from build123d import *

# Parameters (mm, degrees)
CYLINDER189_R               = 5
CYLINDER189_DEPTH           = 8
CYLINDER189_ROLL_ANGLE      = 90
BOX001027045139_W           = 21
BOX001027045139_H           = 10
BOX001027045139_DEPTH       = 28
BOX001027045139_PITCH_ANGLE = 45
BOX001027045138_W           = 21
BOX001027045138_H           = 10
BOX001027045138_DEPTH       = 28
BOX001027045137_W           = 21
BOX001027045137_H           = 8
BOX001027045137_DEPTH       = 28


with BuildPart() as screw_bump_top:
    # Cylinder189 → Cylinder189 (new body)
    with BuildSketch(Plane.XY):
        Circle(CYLINDER189_R)
    extrude(amount=CYLINDER189_DEPTH)


with BuildPart() as screw_bump_top_1:
    # Cylinder189 roll: moved
    add(screw_bump_top.part.rotate(Axis((0, 0, 0), (1, 0, 0)), CYLINDER189_ROLL_ANGLE))


with BuildPart() as screw_bump_top_2:
    # Cylinder189 placement: moved
    add(screw_bump_top_1.part.moved(Location((-6, 0, -1))))


with BuildPart() as cube192:
    # Box001027045139 → Box001027045139 (new body)
    with BuildSketch(Plane.XY):
        with Locations((10.5, 5)):
            Rectangle(BOX001027045139_W, BOX001027045139_H)
    extrude(amount=BOX001027045139_DEPTH)


with BuildPart() as cube192_1:
    # Box001027045139 pitch: moved
    add(cube192.part.rotate(Axis((0, 0, 0), (0, 1, 0)), BOX001027045139_PITCH_ANGLE))


with BuildPart() as cube192_2:
    # Box001027045139 placement: moved
    add(cube192_1.part.moved(Location((-6, -9, 21))))


with BuildPart() as fusion112087:
    # Box001027045138 → Box001027045138 (new body)
    with BuildSketch(Plane(origin=(-6, -9, -7), x_dir=(1, 0, 0), z_dir=(0, 0, 1))):
        with Locations((10.5, 5)):
            Rectangle(BOX001027045138_W, BOX001027045138_H)
    extrude(amount=BOX001027045138_DEPTH)

    # Fusion112087: union Cube192
    add(cube192_2.part)


with BuildPart() as fusion112087_1:
    # Fusion112087 placement: moved
    add(fusion112087.part.moved(Location((10, 0, -17))))


with BuildPart() as top_ghost:
    # Box001027045137 → Box001027045137 (new body)
    with BuildSketch(Plane(origin=(-6, -8, -7), x_dir=(1, 0, 0), z_dir=(0, 0, 1))):
        with Locations((10.5, 4)):
            Rectangle(BOX001027045137_W, BOX001027045137_H)
    extrude(amount=BOX001027045137_DEPTH)

    # Cut160: cut Fusion112087
    add(fusion112087_1.part, mode=Mode.SUBTRACT)

    # Fusion112089: union screw-bump-top
    add(screw_bump_top_2.part)


with BuildPart() as top_ghost_1:
    # Fusion112089 placement: moved
    add(top_ghost.part.moved(Location((0, 0, 28))))


solid = top_ghost_1.part
Design review of the part built by this model. Coordinates are the model's own, in mm. A direction names the side the tool comes from. Coordinates: 2 decimals unless noted, no trailing zeros. Loops run counter-clockwise (first coordinate to the right, second up) from the corner with the lowest first, then second, coordinate; pieces in that order, holes last. Notation, with made-up numbers: (5, -36.75) - (31, -36.75) arc R21 cw to (31, -15.75) - close; hole circle Ø2 at (49, -30.75). An arc over 180 degrees is marked (long way). Use CSV: the item, a comma, the result in double quotes. Start each with the question number.
1. For faces 1 (the flat face through (4, -4, 26)), 2 (the flat face through (4, -4, 49)), 3 (the flat face through (-6, -4, 40)), 4 (the flat face through (-6, -4.1, 21.5)), 5 (the flat face through (-1, -4, 21)), list the 3-axis set-ups (+Z, -Z, +X, -X, +Y, -Y) from which the entire face can be reached by the end or side of a thin tool; tool diameter is ignored.
2. Clearance check with flat-ended pins moving along their axes: pin 1 (2 mm diameter, centred on y = -4, z = 40, fed in from +X); pin 2 (4 mm diameter, centred on y = -2, z = 28, fed in from +X); pin 3 (2.5 mm diameter, centred on y = -5, z = 42.5, fed in from -X). State where each tip first meets the part, or that it passes through.
3. Add section A-A on y = -6. Give the boundary of the cut face in (x, z).
4. Add section B-B on z = 33. Give the boundary of the cut face in (x, y), plus the area to 3 significant figures.
5. To check wall thickness, follow probe 1 along X at (y, z) = (-1, 43); probe 2 along Z at (x, y) = (6.25, -7); probe 3 along X at (y, z) = (-5, 38). State the ranges of each line that lie inside material, in increasing order.
6. Add section C-C on x = 6.5. Give the boundary of the cut face in (y, z).
Resolved:
1,face 1,"-Z, +X, +Y, -Y"
1,face 2,"+Z, +X, -X, +Y, -Y"
1,face 3,"+Z, -X, +Y, -Y"
1,face 4,"-Z, -X, +Y, -Y"
1,face 5,"-Z, +X, -X, +Y, -Y"
2,pin 1,"x = 13"
2,pin 2,"x = 4"
2,pin 3,"x = -6"
3,outline,"(-6, 21) - (4, 21) - (4, 32) - (15, 43) - (15, 49) - (-6, 49) - (-6, 32) arc R5 ccw to (-6, 22) - close"
4,outline,"(-6, -8) - (5, -8) - (5, 0) - (-6, 0) - close"
4,area,"88.0 mm2"
5,probe 1,"-6 to 15"
5,probe 2,"34.25 to 49"
5,probe 3,"-6 to 10"
6,outline,"(-8, 34.5) - (0, 34.5) - (0, 49) - (-8, 49) - close"
